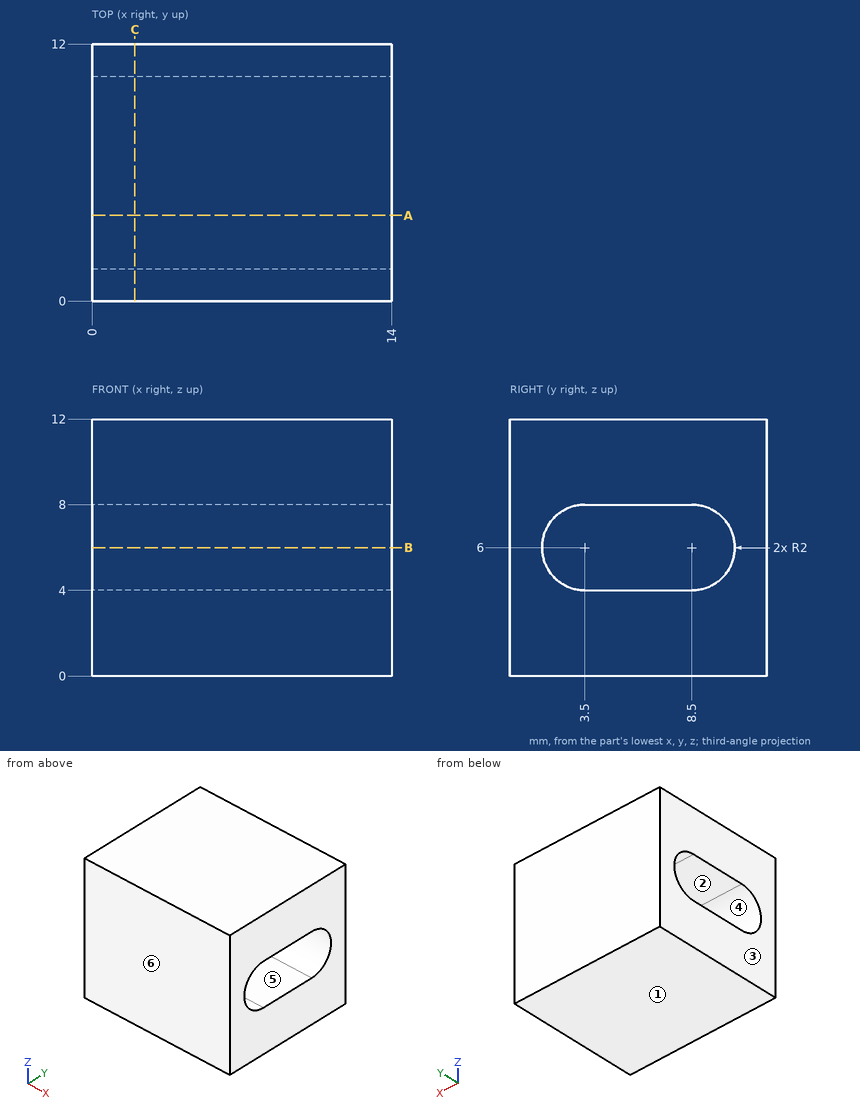
Source: three-view drawing plus pictorial views. Frame: mm from the lowest corner of the part. A direction names the side the tool comes from. Round coordinates to 2 decimals unless told otherwise and drop trailing zeros. Order: outer loops, then holes, each group sorted by start corner. A loop starts at its lowest first (then second) coordinate and runs counter-clockwise, first axis right, second up. Notation, with made-up numbers: (-31.5, 7.25) - (0.5, 7.25) arc R14 ccw to (0.5, 14.25) - close; hole circle Ø4 at (85, -38). An arc over 180 degrees is marked (long way). Use a Markdown table: item, result.
1. Section B-B on z = 6. Return the cut outline in (x, y), then the cut area to 3 significant figures.
Evaluation:
| item | result |
|---|---|
| outline | (0, 0) - (14, 0) - (14, 1.5) - (0, 1.5) - close; (0, 10.5) - (14, 10.5) - (14, 12) - (0, 12) - close |
| area | 42.0 mm^2 |
2. Mould query, pull axis Y, two halves, no side actions, for the marked faces 3, 4, 5 and 6. Classes: +Y half, -Y half, draft (parallel to the pull), parting line (faces both ways), or undercut.
Evaluation:
| item | result |
|---|---|
| face 3 | draft |
| face 4 | undercut |
| face 5 | undercut |
| face 6 | -Y half |
3. Section A-A on y = 4. Return the cut outline in (x, z).
Evaluation:
| item | result |
|---|---|
| outline | (0, 0) - (14, 0) - (14, 4) - (0, 4) - close; (0, 8) - (14, 8) - (14, 12) - (0, 12) - close |
4. Material intervals for probe 1 along Z at (x, y) = (5.25, 4); probe 2 along Z at (x, y) = (13.5, 2.5), sorted ascending.
Evaluation:
| item | result |
|---|---|
| probe 1 | 0 to 4, 8 to 12 |
| probe 2 | 0 to 4.27, 7.73 to 12 |
5. Access query for the marked faces 1 and 2. Directions: +Z, -Z, +X, -X, +Y, -Y. A direction counts if a zero-diameter tool reaches every point of the face in a straight line with its end or side. Return the directions, or none.
Evaluation:
| item | result |
|---|---|
| face 1 | -Z, +X, -X, +Y, -Y |
| face 2 | +X, -X |
6. Section C-C on x = 2. Return the cut outline in (y, z), then the cut area to 3 significant figures.
Evaluation:
| item | result |
|---|---|
| outline | (0, 0) - (12, 0) - (12, 12) - (0, 12) - close; hole (3.5, 4) - (8.5, 4) arc R2 ccw to (8.5, 8) - (3.5, 8) arc R2 ccw to start |
| area | 111 mm^2 |
